Print and shaded views of the part. All mm, measured from the part's lowest x, y and z. A direction names the side the tool comes from. Coordinates: 2 decimals unless noted, no trailing zeros. Write each loop counter-clockwise with the first axis right and the second up, starting at its lowest first coordinate (ties: lowest second). Pieces come first, ordered by that corner, then holes. Notation, with made-up numbers: (-38, -1) -> (-4, -1) arc R9 cw to (-4, 8) -> close; hole circle Ø4 at (-18.5, -37.5). An arc over 180 degrees is marked (long way). Write item = value, one per line.
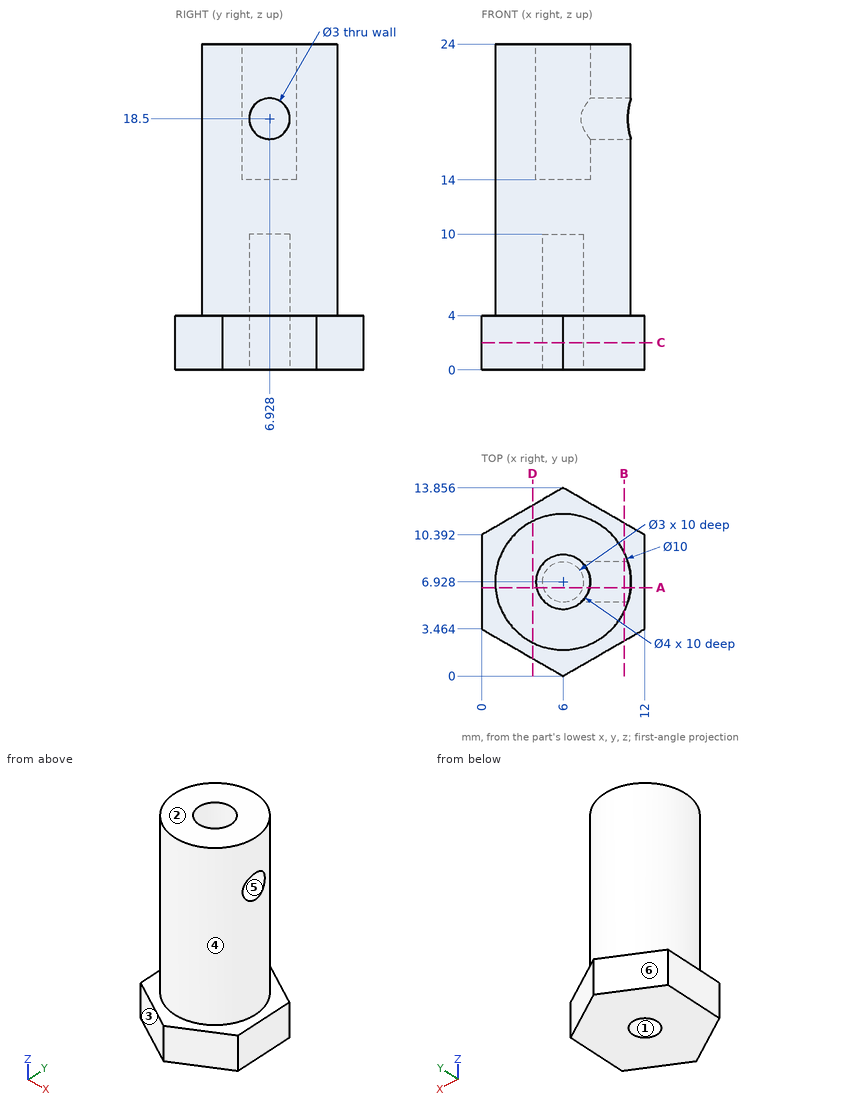
Q1. Probe line 1 (Y direction, x = 6, z = 6); line 2 (Y direction, x = 6, z = 22.25); line 3 (X direction, y = 6, z = 20). List the from-to ranges inside material, lowest first. Write a range as from..to.
Model answer:
line_1 = 1.93..5.43, 8.43..11.93
line_2 = 1.93..4.93, 8.93..11.93
line_3 = 1.09..4.23, 7.77..10.91
Q2. Which spindle directions (+Z, -Z, +X, -X, +Y, -Y) get a long thin tool onto all of the face, cutting with end or side? Do the marked faces 4, 5 and 6. Say none if no direction does.
Model answer:
face_4 = +Z
face_5 = +X
face_6 = +Z, -Z, -X, +Y
Q3. Saw through at D-D on x = 3.75. Give the cut face in (y, z).
Model answer:
outline = (1.3, 0) -> (12.56, 0) -> (12.56, 4) -> (11.39, 4) -> (11.39, 24) -> (2.46, 24) -> (2.46, 4) -> (1.3, 4) -> close
Q4. Pin check, flat tips, straight feed: pin 1 (1.5 mm diameter, centred on x = 6, y = 7, fed in from -Z); pin 2 (2.5 mm diameter, centred on y = 6.93, z = 18.5, fed in from -X); pin 3 (1.5 mm diameter, centred on x = 5, z = 15, fed in from +Y). Stop position of each tip, or through.
Model answer:
pin_1 = 10
pin_2 = 1
pin_3 = 11.92
Q5. Mould opens along X. For the marked faces 1, 2 and 3 say: released by +X, released by -X, zero draft, split by the parting line, or undercut.
Model answer:
face_1 = undercut
face_2 = zero draft
face_3 = released by -X
Q6. Saw through at B-B on x = 10.5. Give the cut face in (y, z), and give its area (3 significant figures).
Model answer:
outline = (2.6, 0) -> (11.26, 0) -> (11.26, 4) -> (9.11, 4) -> (9.11, 24) -> (4.75, 24) -> (4.75, 4) -> (2.6, 4) -> close; hole circle Ø3 at (6.93, 18.5)
area = 115 mm²
Q7. Saw through at A-A on y = 6.5. Give the cut face in (x, z), and give its area (3 significant figures).
Model answer:
outline = (0, 0) -> (4.56, 0) -> (4.56, 10) -> (7.44, 10) -> (7.44, 0) -> (12, 0) -> (12, 4) -> (10.98, 4) -> (10.98, 17.06) -> (7.95, 17.06) -> (7.95, 14) -> (4.05, 14) -> (4.05, 24) -> (1.02, 24) -> (1.02, 4) -> (0, 4) -> close; (7.95, 19.94) -> (10.98, 19.94) -> (10.98, 24) -> (7.95, 24) -> close
area = 171 mm²
Q8. Saw through at C-C on z = 2. Give the cut face in (x, y).
Model answer:
outline = (0, 3.46) -> (6, 0) -> (12, 3.46) -> (12, 10.39) -> (6, 13.86) -> (0, 10.39) -> close; hole circle Ø3 at (6, 6.93)
